from build123d import *

# Parameters (mm, degrees)
SKETCH1_W           = 152.4
SKETCH1_H           = 12.7
BOSS_EXTRUDE1_DEPTH = 2.54
BOSS_EXTRUDE2_DEPTH = 2.54
SKETCH3_R           = 4.445
BOSS_EXTRUDE3_DEPTH = 25.4


with BuildPart() as part:
    # Sketch1 → Boss-Extrude1 (new body)
    with BuildSketch(Plane(origin=(0, 0, 0), x_dir=(1, 0, 0), z_dir=(0, 1, 0))):
        Rectangle(SKETCH1_W, SKETCH1_H)
    extrude(amount=BOSS_EXTRUDE1_DEPTH)

    # Sketch2 → Boss-Extrude2 (add)
    with BuildSketch(Plane(origin=(0, 0, 0), x_dir=(1, 0, 0), z_dir=(0, 1, 0))):
        with BuildLine():
            Line((88.9, 14.199031657), (107.95, 14.199031657))
            Line((107.95, 14.199031657), (146.163989052, -1.529369001))
            ThreePointArc((146.163989052, -1.529369001), (155.312787944, -9.011867032), (158.75, -20.32))
            Line((158.75, -20.32), (158.75, -64.77))
            ThreePointArc((158.75, -64.77), (142.538163249, -94.54763265), (146.05, -128.27))
            ThreePointArc((146.05, -128.27), (119.860653201, -184.91728638), (69.85, -222.25))
            ThreePointArc((69.85, -222.25), (67.089486, -157.7353271), (50.8, -95.25))
            Line((50.8, -95.25), (76.2, -6.35))
            Line((76.2, -6.35), (76.2, 6.35))
            ThreePointArc((76.2, 6.35), (81.435127296, 12.078417757), (88.9, 14.199031657))
        make_face()
    boss_extrude2 = extrude(amount=BOSS_EXTRUDE2_DEPTH)

    # Mirror1: Boss-Extrude2 across plane
    add(boss_extrude2.mirror(Plane(origin=(0, 0, 0), x_dir=(0, 0, 1), z_dir=(1, 0, 0))))

    # Sketch3 → Boss-Extrude3 (add)
    with BuildSketch(Plane.XZ):
        with Locations((88.9, 0)):
            Circle(SKETCH3_R)
        with Locations((138.43, 20.32)):
            Circle(SKETCH3_R)
        with Locations((138.43, 45.72)):
            Circle(SKETCH3_R)
        with Locations((-138.43, 45.72)):
            Circle(SKETCH3_R)
        with Locations((-138.43, 20.32)):
            Circle(SKETCH3_R)
        with Locations((-88.9, 0)):
            Circle(SKETCH3_R)
    extrude(amount=BOSS_EXTRUDE3_DEPTH)


solid = part.part
Geometry: final body of the model. Coordinates: model frame, mm. A direction names the side the tool comes from. Give positions to 0.01 mm unless a question says otherwise; leave off trailing zeros. Order: outer loops, then holes, each group sorted by start corner. A loop starts at its lowest first (then second) coordinate and runs counter-clockwise, first axis right, second up. Notation, with made-up numbers: (13, 72) -> (18, 72) arc R11 cw to (18, 90) -> close; hole circle Ø1 at (-30.75, 54). An arc over 180 degrees is marked (long way). Put each result on its own line as item: value.
Q1. Draft query along X for faces 6 (the face through (155.219, 1.252, 8.873)), 7 (the face through (-63.322, 1.252, 51.422)), 8 (the face through (-126.789, 1.252, -6.445)). Return one class per face: released by +X, released by -X, zero draft, split by the parting line, or undercut.
Here are the results:
face 6: released by +X
face 7: undercut
face 8: released by -X
Q2. Pin query (flat end, axial travel): pin 1 (2 mm diameter, centred on x = 18, y = 1.5, fed in from +Z); pin 2 (1.3 mm diameter, centred on x = -10.5, y = 2, fed in from -Z); pin 3 (6 mm diameter, centred on x = -104, z = 130, fed in from -Y). Return the tip coordinate at first contact, or that it passes through.
Here are the results:
pin 1: stops at z = 6.35
pin 2: stops at z = -6.35
pin 3: stops at y = 0
Q3. Reachability of faces 1 (the face through (-81.34, 1.25, -12.02)), 2 (the face through (67.223, 1.252, 158.631)), 3 (the face through (-84.794, -12.522, -1.702)), 4 (the face through (-155.219, 1.252, 8.873)), 5 (the face through (89, -25.4, 0)) from +Z, -Z, +X, -X, +Y, -Y: full face, straight path, thin tool, end or side. Return the list, or none.
Here are the results:
face 1: -Z, +Y, -Y
face 2: +Y, -Y
face 3: -Y
face 4: -Z, -X, +Y, -Y
face 5: +Z, -Z, +X, -X, -Y
Q4. Material intervals for L1, parallel to Y at x = -133, z = 3; L2, parallel to X at y = -9, z = 43; L3, parallel to Z at x = 142.5, y = -22, sorted ascending.
Here are the results:
L1: y = 0 to 2.54
L2: x = -141.95 to -134.91, 134.91 to 141.95
L3: z = 18.53 to 22.11, 43.93 to 47.51
Q5. Section B-B, the plane x = -37. Return loops of the section in (y, z).
Here are the results:
outline: (0, -6.35) -> (2.54, -6.35) -> (2.54, 6.35) -> (0, 6.35) -> close
Q6. Section A-A, the plane y = -9. Return loops of the section in (x, z) (3 decimals).
Here are the results:
outline: circle Ø8.89 at (-138.43, 20.32); circle Ø8.89 at (-138.43, 45.72); circle Ø8.89 at (-88.9, 0); circle Ø8.89 at (88.9, 0); circle Ø8.89 at (138.43, 20.32); circle Ø8.89 at (138.43, 45.72)
